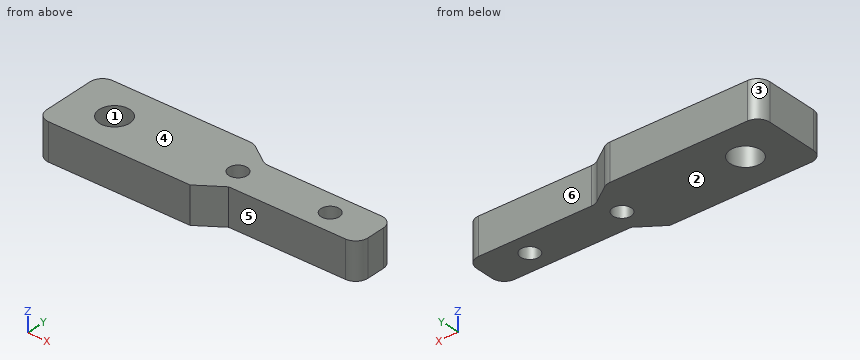
from build123d import *

# Parameters (mm, degrees)
BOSS_EXTRU_1_DEPTH      = 6
ESQUISSE2_R             = 2.5
ESQUISSE2_R_2           = 1.5
ENL_V_MAT_EXTRU_1_DEPTH = 29.298078094
CONG_2_R                = 2


with BuildPart() as part:
    # Esquisse1 → Boss.-Extru.1 (new body)
    with BuildSketch(Plane.XY):
        Polygon((5.939167095, 3.5), (26.939167095, 3.5), (26.939167095, -3.5), (5.939167095, -3.5), (1.939167095, -6.25), (-23.060832905, -6.25), (-23.060832905, 6.25), (1.939167095, 6.25), align=None)
    extrude(amount=BOSS_EXTRU_1_DEPTH)

    # Esquisse2 → Enlèv. mat.-Extru.1 (cut, through all)
    with BuildSketch(Plane.XY.offset(6)):
        with Locations((-15.560832905, 0)):
            Circle(ESQUISSE2_R)
        with Locations((4.539167095, 0)):
            Circle(ESQUISSE2_R_2)
        with Locations((19.539167095, 0)):
            Circle(ESQUISSE2_R_2)
    extrude(amount=-ENL_V_MAT_EXTRU_1_DEPTH, mode=Mode.SUBTRACT)

    # Congé2
    cong_2_edges = [part.edges().sort_by_distance(p)[0] for p in [
        (-23.060832905, 6.25, 3),
        (1.939167095, 6.25, 3),
        (5.939167095, 3.5, 3),
        (26.939167095, 3.5, 3),
        (26.939167095, -3.5, 3),
        (-23.060832905, -6.25, 3),
    ]]
    fillet(cong_2_edges, radius=CONG_2_R)


solid = part.part
Work out the finished part from the listing and answer in its coordinate system (mm). Face numbers are marked on the shaded views. A direction names the side the tool comes from. Give positions to 0.01 mm unless a question says otherwise; leave off trailing zeros. Order: outer loops, then holes, each group sorted by start corner. A loop starts at its lowest first (then second) coordinate and runs counter-clockwise, first axis right, second up. Notation, with made-up numbers: M 39,-11 L 98,-11 A7 cw 98,0 Z; hole C 22.5,-7 d1. An arc over 180 degrees is marked long. Return JSON: item names as keys, results as strings.
Q1. Find section B-B, the plane z = 4.25. Write down the section's boundary in (x, y).
Answer below:
{"outline": "M -23.06,-4.25 A2 ccw -21.06,-6.25 L 1.94,-6.25 L 5.94,-3.5 L 24.94,-3.5 A2 ccw 26.94,-1.5 L 26.94,1.5 A2 ccw 24.94,3.5 L 6.56,3.5 A2 cw 5.43,3.85 L 2.45,5.9 A2 ccw 1.32,6.25 L -21.06,6.25 A2 ccw -23.06,4.25 Z; hole C -15.56,0 d5; hole C 4.54,0 d3; hole C 19.54,0 d3"}
Q2. Find section A-A, the plane y = 0. Write down the section's boundary in (x, z), and give its area (3 significant figures).
Answer below:
{"outline": "M -23.06,0 L -18.06,0 L -18.06,6 L -23.06,6 Z; M -13.06,0 L 3.04,0 L 3.04,6 L -13.06,6 Z; M 6.04,0 L 18.04,0 L 18.04,6 L 6.04,6 Z; M 21.04,0 L 26.94,0 L 26.94,6 L 21.04,6 Z", "area": "234 mm^2"}
Q3. The mould has two halves that part along Y. Classify the marked faces 1, 2 and 3: pulls with the +Y half, pulls with the -Y half, needs draft (parallel to the pull), parting line crosses it, or undercut.
Answer below:
{"face 1": "undercut", "face 2": "needs draft", "face 3": "pulls with the +Y half"}
Q4. Which of the six approach directions +Z, -Z, +X, -X, +Y, -Y give full straight-line access (tool end or side, diameter ignored) to the marked faces 4, 5 and 6?
Answer below:
{"face 4": "+Z, +X, -X, +Y, -Y", "face 5": "+Z, -Z, +X, -Y", "face 6": "+Z, -Z, +X, +Y"}
Q5. Each of these flat-tipped pins is pushed along its axis until it touches: pin 1 (1.5 mm diameter, centred on x = 5, z = 4.5, fed in from +Y); pin 2 (3 mm diameter, centred on x = 21, z = 2, fed in from +Y). Where does it stop, or does it pass through?
Answer below:
{"pin 1": "stops at y = 4.66", "pin 2": "stops at y = 3.5"}
Q6. Find the intervals of material crossed by line 1 along X through (y, z) = (-0.5, 4.55); line 2 along Y through (x, z) = (23.5, 4.1); line 3 along Y through (x, z) = (-13.5, 3), in increasing order. Write a range as [from, to].
Answer below:
{"line 1": "x = [-23.06, -18.01], [-13.11, 3.12], [5.95, 18.12], [20.95, 26.94]", "line 2": "y = [-3.5, 3.5]", "line 3": "y = [-6.25, -1.42], [1.42, 6.25]"}
Q7. Find section C-C, the plane x = 11. Write down the section's boundary in (y, z).
Answer below:
{"outline": "M -3.5,0 L 3.5,0 L 3.5,6 L -3.5,6 Z"}
